Verification items for the finished model (mm, model axes). A direction names the side the tool comes from. Give positions to 0.01 mm unless a question says otherwise; leave off trailing zeros. Order: outer loops, then holes, each group sorted by start corner. A loop starts at its lowest first (then second) coordinate and runs counter-clockwise, first axis right, second up.
from build123d import *

# Parameters (mm, degrees)
F0_R     = 5
F1_DEPTH = 10


# Not quite as in the source:
# - ends of sketch curves that miss each other by under 0.0002 mm in the source are joined


with BuildPart() as f1:
    # F0 (on Top) → F1 (new body)
    with BuildSketch(Plane.XY):
        with BuildLine():
            ThreePointArc((-30.0000003377, 9.9974011055), (-30.0000000844, 9.9987005527), (-30, 10))
            ThreePointArc((-30, 10), (-32.9289321881, 17.0710678119), (-40, 20))
            ThreePointArc((-40, 20), (-47.0719866001, 2.9298510958), (-30.0000003377, 9.9974011055))
        make_face()
        with Locations((-40, 10)):
            Circle(F0_R, mode=Mode.SUBTRACT)
        with BuildLine():
            ThreePointArc((-40, 20), (-32.9289321881, 17.0710678119), (-30, 10))
            ThreePointArc((-30, 10), (-28.8260746289, 12.8286475986), (-25.9963610747, 14))
            Line((-25.9963610747, 14), (20, 14))
            ThreePointArc((20, 14), (24, 10), (20, 6))
            Line((20, 6), (0, 6))
            add(Edge.make_bspline(
                [(0, 0), (-18.0512891521, 0), (-23.9813730686, 0.6377710425), (-18.8085221866, 5.3625723562), (-11.4536762775, 6.3679885575), (-6.8766033776, 5.7466003341), (0, 6)],
                knots=[0, 0, 0, 0, 0.3683888151, 0.5191562868, 0.7199539542, 1, 1, 1, 1], degree=3))
            Line((0, 0), (20, 0))
            ThreePointArc((20, 0), (30, 10), (20, 20))
            Line((20, 20), (-40, 20))
        make_face()
    extrude(amount=F1_DEPTH)


solid = f1.part
(1) Section check D-D, the plane y = 18.75. Enter the section's corners in (x, z).
Solved:
outline: (-44.84, 0) - (24.84, 0) - (24.84, 10) - (-44.84, 10) - close
(2) Section check B-B, the plane y = 9. Enter the section's corners in (x, z), then the cut area to 3 significant figures.
Solved:
outline: (-49.95, 0) - (-44.9, 0) - (-44.9, 10) - (-49.95, 10) - close; (-35.1, 0) - (-30.05, 0) - (-30.05, 10) - (-35.1, 10) - close; (23.87, 0) - (29.95, 0) - (29.95, 10) - (23.87, 10) - close
area: 162 mm2
(3) Scan lines: line 1 (Y direction, x = -40, z = 2.5); line 2 (Y direction, x = 2, z = 5.5); line 3 (Y direction, x = -25, z = 9.25). Record each from-to range of solid material in increasing order.
Solved:
line 1: y = 0 to 5, 15 to 20
line 2: y = 0 to 6, 14 to 20
line 3: y = 14 to 20
(4) Section check A-A, the plane x = 15.5. Enter the section's corners in (y, z).
Solved:
outline: (0, 0) - (6, 0) - (6, 10) - (0, 10) - close; (14, 0) - (20, 0) - (20, 10) - (14, 10) - close
(5) Release check for a two-part mould opening along Y. For faces 4 (the flat face through (10, 0, 5)), 5 (the flat face through (10, 6, 5)), 6 (the flat face through (-10, 20, 5)) record: pulls with the +Y half, pulls with the -Y half, needs draft (parallel to the pull), parting line crosses it, or undercut.
Solved:
face 4: pulls with the -Y half
face 5: undercut
face 6: pulls with the +Y half
(6) Section check C-C, the plane x = -33.5. Enter the section's corners in (y, z), then the cut area to 3 significant figures.
Solved:
outline: (2.4, 0) - (20, 0) - (20, 10) - (2.4, 10) - close
area: 176 mm2
(7) Go/stop test with a flat-tipped pin: pin 1 (2 mm diameter, centred on y = 5.5, z = 4, fed in from -X). Record where the tip stops, or that it passes through.
Solved:
pin 1: stops at x = -49.37
(8) Set-up check for faces 1 (the cylindrical face through (30, 10, 5)), 2 (the cylindrical face through (-28.857, 12.797, 4.93)), 3 (the flat face through (-3, 14, 5)): record each of +Z, -Z, +X, -X, +Y, -Y from which the full face is reachable in a straight line by a thin tool's end or side.
Solved:
face 1: +Z, -Z, +X
face 2: +Z, -Z, -Y
face 3: +Z, -Z
